from build123d import *

# Parameters (mm, degrees)
F1_DEPTH  = 7
F3_DEPTH  = 25
F5_DEPTH  = 25
F7_DEPTH  = 25
F8_W      = 20
F8_H      = 59.9582853711
F8_H_2    = 57.0417146289
F9_DEPTH  = 3.7
F11_DEPTH = 3.7


with BuildPart() as f1:
    # F0 (on Top) → F1 (new body)
    with BuildSketch(Plane.XY):
        with BuildLine():
            Line((177.6268834546, 63.9582853711), (-95.3731165454, 63.9582853711))
            ThreePointArc((-95.3731165454, 63.9582853711), (-98.9086504513, 62.493819277), (-100.3731165454, 58.9582853711))
            Line((-100.3731165454, 58.9582853711), (-100.3731165454, -56.0417146289))
            ThreePointArc((-100.3731165454, -56.0417146289), (-98.9086504513, -59.5772485349), (-95.3731165454, -61.0417146289))
            Line((-95.3731165454, -61.0417146289), (177.6268834546, -61.0417146289))
            Line((177.6268834546, -61.0417146289), (177.6268834546, 63.9582853711))
        make_face()
    extrude(amount=F1_DEPTH)

    # F2 (on face) → F3 (cut)
    with BuildSketch(Plane.XY.offset(7)):
        with BuildLine():
            Line((177.6268834546, -4), (177.6268834546, 0))
            Line((177.6268834546, 0), (0, 0))
            ThreePointArc((0, 0), (1.1715728753, -2.8284271247), (4, -4))
            Line((4, -4), (177.6268834546, -4))
        make_face()
    extrude(amount=-F3_DEPTH, mode=Mode.SUBTRACT)

    # F4 (on face) → F5 (cut)
    with BuildSketch(Plane.XY.offset(7)):
        with BuildLine():
            ThreePointArc((4, 4), (1.1715728753, 2.8284271247), (0, 0))
            Line((0, 0), (177.6268834546, 0))
            Line((177.6268834546, 0), (177.6268834546, 4))
            Line((177.6268834546, 4), (4, 4))
        make_face()
    extrude(amount=-F5_DEPTH, mode=Mode.SUBTRACT)

    # F6 (on face) → F7 (cut)
    with BuildSketch(Plane.XY.offset(7)):
        with BuildLine():
            ThreePointArc((-100.3731165454, -7.9999726506), (-94.7027443402, -5.6642452842), (-92.3521978855, 0))
            ThreePointArc((-92.3521978855, 0), (-94.7027443402, 5.6642452842), (-100.3731165454, 7.9999726506))
            Line((-100.3731165454, 7.9999726506), (-100.3731165454, -7.9999726506))
        make_face()
    extrude(amount=-F7_DEPTH, mode=Mode.SUBTRACT)

    # F8 (on face) → F9 (cut)
    with BuildSketch(Plane.XY.offset(7)):
        with Locations((167.6268834546, 33.9791426855)):
            Rectangle(F8_W, F8_H)
        with Locations((167.6268834546, -32.5208573145)):
            Rectangle(F8_W, F8_H_2)
    extrude(amount=-F9_DEPTH, mode=Mode.SUBTRACT)

    # F10 (on face) → F11 (cut)
    with BuildSketch(Plane.XY.offset(7)):
        with BuildLine():
            Line((157.6268834546, 43.9582853711), (157.6268834546, 63.9582853711))
            Line((157.6268834546, 63.9582853711), (-95.3731165454, 63.9582853711))
            ThreePointArc((-95.3731165454, 63.9582853711), (-98.9086504513, 62.493819277), (-100.3731165454, 58.9582853711))
            Line((-100.3731165454, 58.9582853711), (-100.3731165454, 43.9582853711))
            Line((-100.3731165454, 43.9582853711), (157.6268834546, 43.9582853711))
        make_face()
        with BuildLine():
            Line((157.6268834546, -41.0417146289), (-100.3731165454, -41.0417146289))
            Line((-100.3731165454, -41.0417146289), (-100.3731165454, -56.0417146289))
            ThreePointArc((-100.3731165454, -56.0417146289), (-98.9086504513, -59.5772485349), (-95.3731165454, -61.0417146289))
            Line((-95.3731165454, -61.0417146289), (157.6268834546, -61.0417146289))
            Line((157.6268834546, -61.0417146289), (157.6268834546, -41.0417146289))
        make_face()
    extrude(amount=-F11_DEPTH, mode=Mode.SUBTRACT)


solid = f1.part
Source: CAD feature listing. Evaluate the final solid. Frame: model axes, mm. Round coordinates to 2 decimals unless told otherwise and drop trailing zeros. Loops run counter-clockwise (first coordinate to the right, second up) from the corner with the lowest first, then second, coordinate; pieces in that order, holes last. Notation, with made-up numbers: (80, 73.5) - (118, 73.5) arc R21 ccw to (118, 100.5) - close; hole circle Ø7 at (54.5, -4.5). An arc over 180 degrees is marked (long way). Write item = value, one per line. Start each with the question number.
(1) Section query A-A, the plane x = 86. Output: boundary loops of the cut face in (y, z), plus the area to 3 significant figures.
(2) Section query C-C, the plane y = -16. Output: boundary loops of the cut face in (x, z), plus the area to 3 significant figures.
(3) Ray query, line 1 along Y through (x, z) = (57, 3); line 2 along Y through (x, z) = (70, 4.5); line 3 along X through (y, z) = (29, 4.5). Return the intervals inside material, ascending. Write a range as from..to.
(4) Pull-direction query (Y, two-part tool) for faces 1 (the face through (92, 4, 4)), 2 (the face through (68, -45, 3.3)), 3 (the face through (90, -4, 4)), 4 (the face through (-98.9, 62.5, 1.6)); classes: +Y half, -Y half, draft (parallel to the pull), parting line (faces both ways), or undercut.
(5) Section query D-D, the plane x = -16.5. Output: boundary loops of the cut face in (y, z).
(6) Pin query (flat end, axial travel): pin 1 (1.1 mm diameter, centred on x = -31, z = 5.5, fed in from +Y); pin 2 (1.8 mm diameter, centred on y = 32, z = 4.5, fed in from +X); pin 3 (8 mm diameter, centred on x = 111.5, y = 21, fed in from -Z); pin 4 (1.8 mm diameter, centred on x = 16.5, z = 5, fed in from -Y). Return the tip coordinate at first contact, or that it passes through.
(7) Section query B-B, the plane z = 1.5. Output: boundary loops of the cut face in (x, y).
Conclusion:
q1.outline = (-61.04, 0) - (-4, 0) - (-4, 7) - (-41.04, 7) - (-41.04, 3.3) - (-61.04, 3.3) - close; (4, 0) - (63.96, 0) - (63.96, 3.3) - (43.96, 3.3) - (43.96, 7) - (4, 7) - close
q1.area = 671 mm2
q2.outline = (-100.37, 0) - (177.63, 0) - (177.63, 3.3) - (157.63, 3.3) - (157.63, 7) - (-100.37, 7) - close
q2.area = 1,870 mm2
q3.line_1 = -61.04..-4, 4..63.96
q3.line_2 = -41.04..-4, 4..43.96
q3.line_3 = -100.37..157.63
q4.face_1 = undercut
q4.face_2 = draft
q4.face_3 = undercut
q4.face_4 = +Y half
q5.outline = (-61.04, 0) - (63.96, 0) - (63.96, 3.3) - (43.96, 3.3) - (43.96, 7) - (-41.04, 7) - (-41.04, 3.3) - (-61.04, 3.3) - close
q6.pin_1 = 43.96
q6.pin_2 = 157.63
q6.pin_3 = 0
q6.pin_4 = -41.04
q7.outline = (-100.37, -56.04) arc R5 ccw to (-95.37, -61.04) - (177.63, -61.04) - (177.63, -4) - (4, -4) arc R4 cw to (4, 4) - (177.63, 4) - (177.63, 63.96) - (-95.37, 63.96) arc R5 ccw to (-100.37, 58.96) - (-100.37, 8) arc R8 cw (long way) to (-100.37, -8) - close
